Geometry: final body of the model. Coordinates: model frame, mm. A direction names the side the tool comes from. Give positions to 0.01 mm unless a question says otherwise; leave off trailing zeros. Order: outer loops, then holes, each group sorted by start corner. A loop starts at its lowest first (then second) coordinate and runs counter-clockwise, first axis right, second up. Notation, with made-up numbers: (78, 25) -> (109, 25) arc R32 ccw to (109, 60) -> close; hole circle Ø4 at (46.25, 17.5). An arc over 180 degrees is marked (long way). One line per item, written item: value. Start each with the question number.
```python
from build123d import *

# Parameters (mm, degrees)
SKETCH1_R           = 1.85
SKETCH1_R_2         = 4
SKETCH1_W           = 27.178
SKETCH1_H           = 12.192
BOSS_EXTRUDE1_DEPTH = 5


with BuildPart() as part:
    # Sketch1 → Boss-Extrude1 (new body)
    with BuildSketch(Plane(origin=(0, 5, 0), x_dir=(1, 0, 0), z_dir=(0, 1, 0))):
        with BuildLine():
            Line((64, 13.5), (0, 13.5))
            ThreePointArc((0, 13.5), (-13.5, 0), (0, -13.5))
            Line((0, -13.5), (64, -13.5))
            ThreePointArc((64, -13.5), (77.5, 0), (64, 13.5))
        make_face()
        with Locations((56, 0)):
            Circle(SKETCH1_R, mode=Mode.SUBTRACT)
        with Locations((64, -8)):
            Circle(SKETCH1_R, mode=Mode.SUBTRACT)
        with Locations((72, 0)):
            Circle(SKETCH1_R, mode=Mode.SUBTRACT)
        with Locations((64, 8)):
            Circle(SKETCH1_R, mode=Mode.SUBTRACT)
        with Locations((64, 0)):
            Circle(SKETCH1_R_2, mode=Mode.SUBTRACT)
        with Locations((-8, 0)):
            Circle(SKETCH1_R, mode=Mode.SUBTRACT)
        with Locations((0, -8)):
            Circle(SKETCH1_R, mode=Mode.SUBTRACT)
        with Locations((8, 0)):
            Circle(SKETCH1_R, mode=Mode.SUBTRACT)
        with Locations((0, 8)):
            Circle(SKETCH1_R, mode=Mode.SUBTRACT)
        Circle(SKETCH1_R_2, mode=Mode.SUBTRACT)
        with Locations((32, 0)):
            Rectangle(SKETCH1_W, SKETCH1_H, mode=Mode.SUBTRACT)
    extrude(amount=-BOSS_EXTRUDE1_DEPTH)


solid = part.part
```
1. Access query for faces 4 (the flat face through (32, 3, -6.096)), 5 (the cylindrical face through (-13.497, 2.535, -0.297)). Directions: +Z, -Z, +X, -X, +Y, -Y. A direction counts if a zero-diameter tool reaches every point of the face in a straight line with its end or side. Return the directions, or none.
2. Cut plane B-B, the plane x = 24. Return loops of the section in (y, z).
3. Cut plane D-D, the plane z = -8. Return loops of the section in (x, y), then the cut area to 3 significant figures.
4. Cut plane A-A, the plane y = 2.85. State how many separate pieces and enclosed holes the cut face has, then the cut area to 3 significant figures.
5. Draft query along Z for faces 1 (the flat face through (32, 3, -13.5)), 2 (the flat face through (31, 0, -9)), 3 (the cylindrical face through (0.854, 2.535, 9.641)). Return one class per face: pulls with the +Z half, pulls with the -Z half, needs draft (parallel to the pull), parting line crosses it, or undercut.
6. Pin query (flat end, axial travel): P1, Ø1.5, axis at x = 56, z = -2, coming from the -Y side. Return the tip coordinate at first contact, or that it passes through.
7. Material intervals for L1, parallel to Z at x = 64, y = 3.7; L2, parallel to X at y = 2.1, z = 8; L3, parallel to X at y = 2.85, z = 9.5, sorted ascending. Write a range as [from, to].
Answers follow:
1. face 4: +Y, -Y
1. face 5: -X, +Y, -Y
2. outline: (0, -13.5) -> (5, -13.5) -> (5, -6.1) -> (0, -6.1) -> close; (0, 6.1) -> (5, 6.1) -> (5, 13.5) -> (0, 13.5) -> close
3. outline: (-10.87, 0) -> (-1.85, 0) -> (-1.85, 5) -> (-10.87, 5) -> close; (1.85, 0) -> (62.15, 0) -> (62.15, 5) -> (1.85, 5) -> close; (65.85, 0) -> (74.87, 0) -> (74.87, 5) -> (65.85, 5) -> close
3. area: 392 mm²
4. separate pieces: 1
4. enclosed holes: 11
4. area: 1,780 mm²
5. face 1: pulls with the -Z half
5. face 2: needs draft
5. face 3: undercut
6. P1: stops at y = 0
7. L1: z = [-13.5, -9.85], [-6.15, -4], [4, 6.15], [9.85, 13.5]
7. L2: x = [-10.87, -1.85], [1.85, 62.15], [65.85, 74.87]
7. L3: x = [-9.59, -1.08], [1.08, 62.92], [65.08, 73.59]
